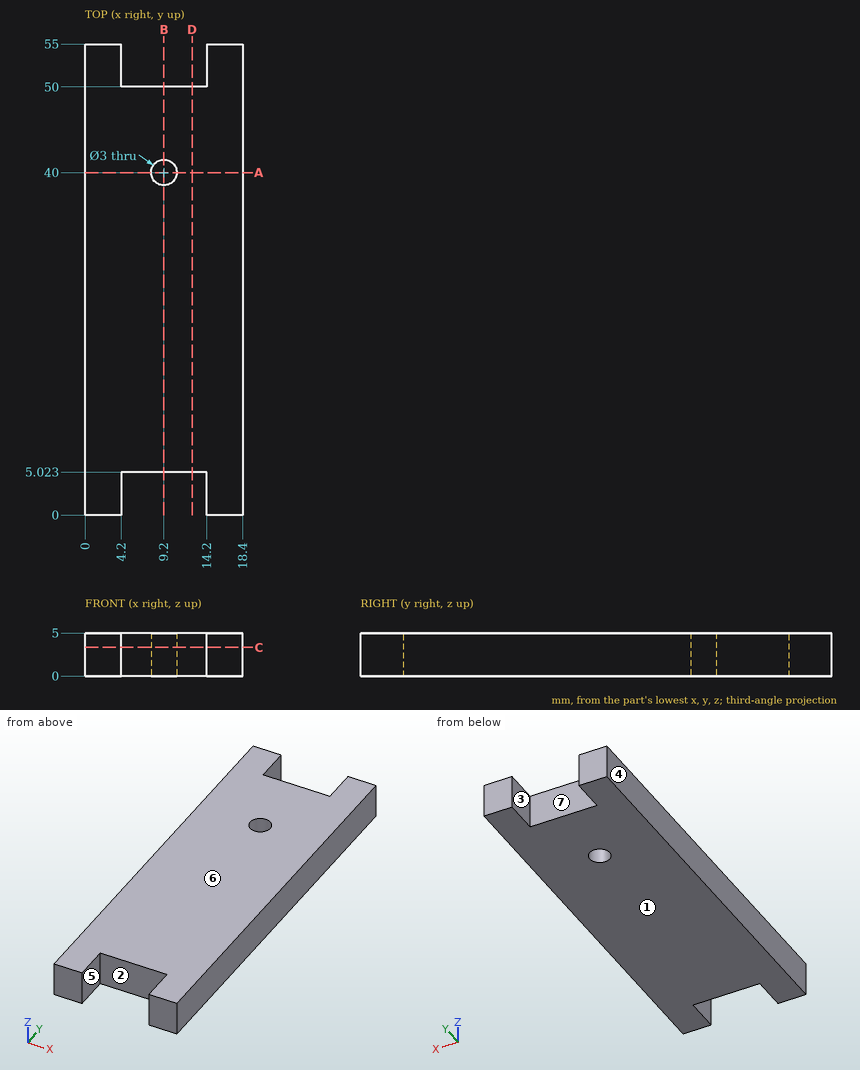
Verification items for this drawing (mm, ordinates from the low corner). A direction names the side the tool comes from. Coordinates: 2 decimals unless noted, no trailing zeros. Order: outer loops, then holes, each group sorted by start corner. A loop starts at its lowest first (then second) coordinate and runs counter-clockwise, first axis right, second up. Notation, with made-up numbers: (33.5, 55.5) -> (77.5, 55.5) arc R24 ccw to (77.5, 93.5) -> close; hole circle Ø3 at (24.25, 1). An arc over 180 degrees is marked (long way). Put each result on its own line as item: value. Start each with the question number.
1. Cross-section at A-A, the plane y = 40. Record the boundary of the cut face in (x, z).
2. Cross-section at B-B, the plane x = 9.2. Record the boundary of the cut face in (y, z), then the cut area to 3 significant figures.
3. Material ranges on L1, parallel to X at y = 40, z = 3.5; L2, parallel to Y at x = 9.2, z = 3.7; L3, parallel to Y at x = 5.75, z = 0.6, recorded low to high. Write a range as [from, to].
4. Access from +Z, -Z, +X, -X, +Y, -Y to the whole of each face (thin tool, end or side, straight path). Record for the marked faces 1, 2 and 3.
5. Cross-section at D-D, the plane x = 12.5. Record the boundary of the cut face in (y, z), then the cut area to 3 significant figures.
6. Go/stop test with flat-tipped pins: pin 1 Ø8 at (x, y) = (7.5, 33.5) entering from -Z; pin 2 Ø1.5 at (x, z) = (8.5, 3) entering from +Y. Record where each tip stops, or that it passes through.
7. Mould release check, pull along X, two halves, no side actions. Record for the marked faces 4, 5, 6 and 7: released by +X, released by -X, zero draft, split by the parting line, or undercut.
8. Cross-section at C-C, the plane z = 3.35. Record the boundary of the cut face in (x, y).
Computed:
1. outline: (0, 0) -> (7.7, 0) -> (7.7, 5) -> (0, 5) -> close; (10.7, 0) -> (18.4, 0) -> (18.4, 5) -> (10.7, 5) -> close
2. outline: (5.02, 0) -> (38.5, 0) -> (38.5, 5) -> (5.02, 5) -> close; (41.5, 0) -> (50, 0) -> (50, 5) -> (41.5, 5) -> close
2. area: 210 mm2
3. L1: [0, 7.7], [10.7, 18.4]
3. L2: [5.02, 38.5], [41.5, 50]
3. L3: [5.02, 50]
4. face 1: -Z, +X, -X, +Y, -Y
4. face 2: +Z, -Z, -Y
4. face 3: +Z, -Z, +Y
5. outline: (5.02, 0) -> (50, 0) -> (50, 5) -> (5.02, 5) -> close
5. area: 225 mm2
6. pin 1: z = 0
6. pin 2: y = 50
7. face 4: released by -X
7. face 5: undercut
7. face 6: zero draft
7. face 7: undercut
8. outline: (0, 0) -> (4.2, 0) -> (4.2, 5.02) -> (14.2, 5.02) -> (14.2, 0) -> (18.4, 0) -> (18.4, 55) -> (14.2, 55) -> (14.2, 50) -> (4.2, 50) -> (4.2, 55) -> (0, 55) -> close; hole circle Ø3 at (9.2, 40)
